```python
from build123d import *

# Parameters (mm, degrees)
SKETCH1_W           = 229.616
SKETCH1_H           = 110.998
BOSS_EXTRUDE1_DEPTH = 12.7
DRAFT1_ANGLE        = -45
CUT_EXTRUDE1_DEPTH  = 139.893248743
CUT_EXTRUDE2_DEPTH  = 139.893248743
CUT_EXTRUDE3_DEPTH  = 139.893248743
SKETCH5_R           = 14.406124238
CUT_EXTRUDE4_DEPTH  = 139.893248743


with BuildPart() as part:
    # Sketch1 → Boss-Extrude1 (new body)
    with BuildSketch(Plane(origin=(0, 0, 0), x_dir=(1, 0, 0), z_dir=(0, 1, 0))):
        with Locations((0, 21.631847801)):
            Rectangle(SKETCH1_W, SKETCH1_H)
    extrude(amount=BOSS_EXTRUDE1_DEPTH)

    # Draft1
    draft1_faces = [part.faces().sort_by_distance(p)[0] for p in [
        (-114.808, 6.35, -21.631847801),
        (114.808, 6.35, -21.631847801),
    ]]
    draft(draft1_faces, Plane.ZX.offset(12.7), DRAFT1_ANGLE)

    # Sketch2 → Cut-Extrude1 (cut, through all)
    with BuildSketch(Plane(origin=(0, 12.7, 0), x_dir=(1, 0, 0), z_dir=(0, 1, 0))):
        with BuildLine():
            Line((-114.808, -9.356152199), (-97.477466366, -9.356152199))
            ThreePointArc((-97.477466366, -9.356152199), (-88.138, -9.356152199), (-88.138, -18.695618565))
            Line((-88.138, -18.695618565), (-88.138, -33.867152199))
            Line((-88.138, -33.867152199), (-114.808, -33.867152199))
            Line((-114.808, -33.867152199), (-114.808, -9.356152199))
        make_face()
        with BuildLine():
            Line((114.808, -33.867152199), (114.808, -9.356152199))
            Line((114.808, -9.356152199), (97.477466366, -9.356152199))
            ThreePointArc((97.477466366, -9.356152199), (88.138, -9.356152199), (88.138, -18.695618565))
            Line((88.138, -18.695618565), (88.138, -33.867152199))
            Line((88.138, -33.867152199), (114.808, -33.867152199))
        make_face()
        with BuildLine():
            Line((-114.808, 58.969847801), (-91.336585113, 58.969847801))
            ThreePointArc((-91.336585113, 58.969847801), (-82.215723928, 60.978708985), (-84.224585113, 70.099570169))
            Line((-84.224585113, 70.099570169), (-84.224585113, 77.130847801))
            Line((-84.224585113, 77.130847801), (-114.808, 77.130847801))
            Line((-114.808, 77.130847801), (-114.808, 58.969847801))
        make_face()
    extrude(amount=-CUT_EXTRUDE1_DEPTH, mode=Mode.SUBTRACT)

    # Sketch3 → Cut-Extrude2 (cut, through all)
    with BuildSketch(Plane(origin=(0, 12.7, 0), x_dir=(1, 0, 0), z_dir=(0, 1, 0))):
        with BuildLine():
            Line((3.048, 41.385190987), (-5.690853499, -3.137191319))
            ThreePointArc((-5.690853499, -3.137191319), (-4.398442962, -8.495486175), (0.508, -11.007152199))
            Line((0.508, -11.007152199), (60.043235464, -13.547152199))
            ThreePointArc((60.043235464, -13.547152199), (64.017965036, -12.423899948), (66.548, -9.159073174))
            Line((66.548, -9.159073174), (86.868, 48.063309133))
            ThreePointArc((86.868, 48.063309133), (85.755892247, 54.455195083), (79.710737995, 56.810847801))
            Line((79.710737995, 56.810847801), (8.59435603, 46.650847801))
            ThreePointArc((8.59435603, 46.650847801), (4.981382787, 44.902582041), (3.048, 41.385190987))
        make_face()
    extrude(amount=-CUT_EXTRUDE2_DEPTH, mode=Mode.SUBTRACT)

    # Sketch4 → Cut-Extrude3 (cut, through all)
    with BuildSketch(Plane.XZ):
        with BuildLine():
            Line((-43.477968603, -77.130847801), (-43.477968603, -58.969847801))
            ThreePointArc((-43.477968603, -58.969847801), (-36.873968603, -52.365847801), (-30.269968603, -58.969847801))
            Line((-30.269968603, -58.969847801), (-11.219968603, -58.969847801))
            ThreePointArc((-11.219968603, -58.969847801), (-4.615968603, -65.573847801), (-11.219968603, -72.177847801))
            Line((-11.219968603, -72.177847801), (-11.219968603, -77.130847801))
            Line((-11.219968603, -77.130847801), (-43.477968603, -77.130847801))
        make_face()
    extrude(amount=-CUT_EXTRUDE3_DEPTH, mode=Mode.SUBTRACT)

    # Sketch5 → Cut-Extrude4 (cut, through all)
    with BuildSketch(Plane.XZ):
        with Locations(Location((-54.2628102, -21.286098046, 0), (0, 0, 270))):
            Circle(SKETCH5_R)
    extrude(amount=-CUT_EXTRUDE4_DEPTH, mode=Mode.SUBTRACT)


solid = part.part
```
Part model, mm, in its own coordinate system. A direction names the side the tool comes from. Round coordinates to 2 decimals unless told otherwise and drop trailing zeros. Order: outer loops, then holes, each group sorted by start corner. A loop starts at its lowest first (then second) coordinate and runs counter-clockwise, first axis right, second up. Notation, with made-up numbers: M -13,37.5 L 39,37.5 A20 ccw 39,68.5 Z; hole C 47,86 d6. An arc over 180 degrees is marked long. Put each result on its own line as item: value. Start each with the question number.
1. Slice it at A-A on z = -24. List the corners of the cut face in (x, y).
2. Drop flat-ended pins along their axis: pin 1 (2 mm diameter, centred on y = 3.5, z = -74.5, fed in from -X); pin 2 (1 mm diameter, centred on x = -42, y = 2, fed in from -Z); pin 3 (2 mm diameter, centred on y = 11, z = -52.5, fed in from -X). Give the stop position or say it passes through.
3. Drill centre lines: probe 1 along X at (y, z) = (4.5, -31); probe 2 along Z at (x, y) = (10.5, 1.5); probe 3 along X at (y, z) = (4, 4). Where is each one in solid material? Low to high. Write a range as [from, to].
4. Tool access for faces 5 (the face through (104, 8, 9.356)), 6 (the face through (-88.138, 6, 26)), 7 (the face through (5.02, 6.44, -44.94)): list every direction of +Z, -Z, +X, -X, +Y, -Y with a clear straight run to the whole face (end or side of a thin tool).
5. Slice it at B-B on x = 51. List the corners of the cut face in (y, z), then the cut area to 3 significant figures.
6. Slice it at C-C on y = 10.25. List the corners of the cut face in (x, z).
7. Two-plate mould, pull along X, no slides. Class faces 1 (the face through (88.138, 6, 26)), 2 (the face through (-64, 6, -77.131)), 3 (the face through (44.65, 6.44, -51.8)), 4 (the face through (-84.225, 6, -74)): +X half, -X half, draft (parallel to the pull), parting line (faces both ways), or undercut.
8. Slice it at D-D on z = -43.5. List the corners of the cut face in (x, y), then the cut area to 3 significant figures.
Findings:
1. outline: M -114.81,12.7 L -102.11,0 L -68.41,0 L -68.41,12.7 Z; M -40.11,0 L -0.36,0 L -0.36,12.7 L -40.11,12.7 Z; M 78.32,0 L 102.11,0 L 114.81,12.7 L 78.32,12.7 Z
2. pin 1: x = -84.22
2. pin 2: z = -55.51
2. pin 3: x = -114.11
3. probe 1: [-106.61, -64.9], [-43.62, 1.01], [80.81, 106.61]
3. probe 2: [-77.13, -46.92], [11.43, 33.87]
3. probe 3: [-106.11, -5.8], [68.38, 106.11]
4. face 5: +Z, +X, +Y, -Y
4. face 6: +Z, -X, +Y, -Y
4. face 7: +Y, -Y
5. outline: M 0,-77.13 L 12.7,-77.13 L 12.7,-52.71 L 0,-52.71 Z; M 0,13.16 L 12.7,13.16 L 12.7,33.87 L 0,33.87 Z
5. area: 573 mm2
6. outline: M -112.36,-58.97 L -91.34,-58.97 A6.6 cw -84.22,-70.1 L -84.22,-77.13 L -43.48,-77.13 L -43.48,-58.97 A6.6 cw -30.27,-58.97 L -11.22,-58.97 A6.6 cw -11.22,-72.18 L -11.22,-77.13 L 112.36,-77.13 L 112.36,9.36 L 97.48,9.36 A6.6 cw 88.14,18.7 L 88.14,33.87 L -88.14,33.87 L -88.14,18.7 A6.6 cw -97.48,9.36 L -112.36,9.36 Z; hole C -54.26,-21.29 d28.81; hole M -5.69,3.14 L 3.05,-41.39 A6.6 ccw 8.59,-46.65 L 79.71,-56.81 A6.6 ccw 86.87,-48.06 L 66.55,9.16 A6.6 ccw 60.04,13.55 L 0.51,11.01 A6.6 ccw Z
7. face 1: +X half
7. face 2: draft
7. face 3: undercut
7. face 4: -X half
8. outline: M -114.81,12.7 L -102.11,0 L 3.86,0 L 3.86,12.7 Z; M 85.25,0 L 102.11,0 L 114.81,12.7 L 85.25,12.7 Z
8. area: 1,720 mm2
